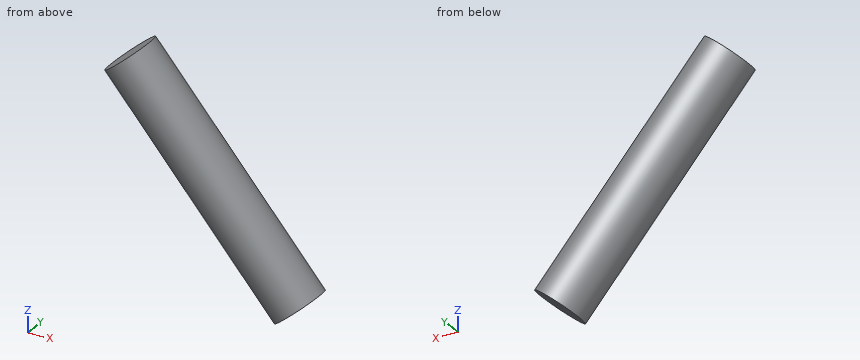
```python
from build123d import *

# Parameters (mm, degrees)
CYLINDER154_R                     = 1.5
CYLINDER154_DEPTH                 = 15
CYLINDER154_PLACEMENT_ANGLE       = 40
PART_MIRRORING002_PLACEMENT_ANGLE = 90


with BuildPart() as cylinder154:
    # Cylinder154 → Cylinder154 (new body)
    with BuildSketch(Plane.XY):
        Circle(CYLINDER154_R)
    extrude(amount=CYLINDER154_DEPTH)


with BuildPart() as cylinder154_1:
    # Cylinder154 placement: moved
    add(cylinder154.part.moved(Location((0, -251.493993, -317.931136))).rotate(Axis((0, -251.493993, -317.931136), (-1, 0, 0)), CYLINDER154_PLACEMENT_ANGLE))


with BuildPart() as part_mirroring002:
    # Part__Mirroring002: instance of Cylinder154
    add(cylinder154_1.part.mirror(Plane(origin=(0, 0, 0), x_dir=(1, 0, 0), z_dir=(0, 1, 0))))


with BuildPart() as part_mirroring002_1:
    # Part__Mirroring002 placement: moved
    add(part_mirroring002.part.moved(Location((291.3, -284.14, 0.98))).rotate(Axis((291.3, -284.14, 0.98), (0, 0, 1)), PART_MIRRORING002_PLACEMENT_ANGLE))


with BuildPart() as part_mirroring003:
    # Part__Mirroring003: instance of Part__Mirroring002
    add(part_mirroring002_1.part.mirror(Plane(origin=(0, 0, 0), x_dir=(0, -1, 0), z_dir=(1, 0, 0))))


solid = part_mirroring003.part
```
Geometry check sheet. Reference: the model listing, model coordinates, mm. Round coordinates to 2 decimals unless told otherwise and drop trailing zeros. Loops run counter-clockwise (first coordinate to the right, second up) from the corner with the lowest first, then second, coordinate; pieces in that order, holes last. Notation, with made-up numbers: (-32.75, 88) - (-25.75, 88) arc R7 cw to (-25.75, 96) - close; hole circle Ø3 at (45, 80.25). An arc over 180 degrees is marked (long way). Write item = value, one per line. Start each with the question number.
1. Depth check by flat-ended pin: pin 1 (1 mm diameter, centred on x = -45.5, y = -283.5, fed in from -Z); pin 2 (1 mm diameter, centred on x = -42, z = -314, fed in from +Y); pin 3 (1 mm diameter, centred on x = -45, z = -313.5, fed in from +Y). Enter the tip coordinate at first touch or a pass-through.
2. Section check A-A on y = -285.35. Enter the section's corners in (x, z), then the cut area to 3 significant figures.
3. Thickness scan on line 1 (Z direction, x = -48.25, y = -284.2); line 2 (Z direction, x = -47.5, y = -283.05); line 3 (X direction, y = -284.05, z = -314). Record the ranges inside material, lowest first.
4. Section check B-B on y = -283. Enter the section's corners in (x, z), then the cut area to 3 significant figures.
Working result:
q1.pin_1 = -312.94
q1.pin_2 = -282.64
q1.pin_3 = -283.33
q2.outline = (-50.13, -306.03) - (-40.49, -317.52) - (-39.13, -316.38) - (-48.77, -304.89) - close
q2.area = 26.6 mm^2
q3.line_1 = -309.22 to -304.56
q3.line_2 = -309.38 to -306.18
q3.line_3 = -44.24 to -40.33
q4.outline = (-50.19, -306.09) - (-40.55, -317.58) - (-39.06, -316.32) - (-48.7, -304.83) - close
q4.area = 29.2 mm^2
